```python
from build123d import *

# Parameters (mm, degrees)
F1_DEPTH = 152.4


# Not quite as in the source:
# - ends of sketch curves that miss each other by under 0.0002 mm in the source are joined


with BuildPart() as f1:
    # F0 (on Front) → F1 (new body)
    with BuildSketch(Plane.XZ):
        with BuildLine():
            Line((-8.73125, 3.7119814), (-8.73125, 0.9179814))
            Line((-8.73125, 0.9179814), (-3.96875, 0.9179814))
            Line((-3.96875, 0.9179814), (-3.96875, -7.0195186))
            Line((-3.96875, -7.0195186), (8.73125, -7.0195186))
            Line((8.73125, -7.0195186), (8.73125, -2.0665186))
            ThreePointArc((8.73125, -2.0665186), (5.7032908876, -1.3612616552), (4.438258034, 1.4787376653))
            ThreePointArc((4.438258034, 1.4787376653), (4.3678620463, 1.6652468114), (4.1844976, 1.7434814))
            Line((4.1844976, 1.7434814), (2.06375, 1.7434814))
            ThreePointArc((2.06375, 1.7434814), (1.1469309524, 3.8652258573), (-0.1916191114, 5.7495426677))
            ThreePointArc((-0.1916191114, 5.7495426677), (-4.0073604602, 6.8451953761), (-6.4452349512, 3.7119803958))
            Line((-6.4452349512, 3.7119803958), (-8.73125, 3.7119814))
        make_face()
    extrude(amount=F1_DEPTH)


solid = f1.part
```
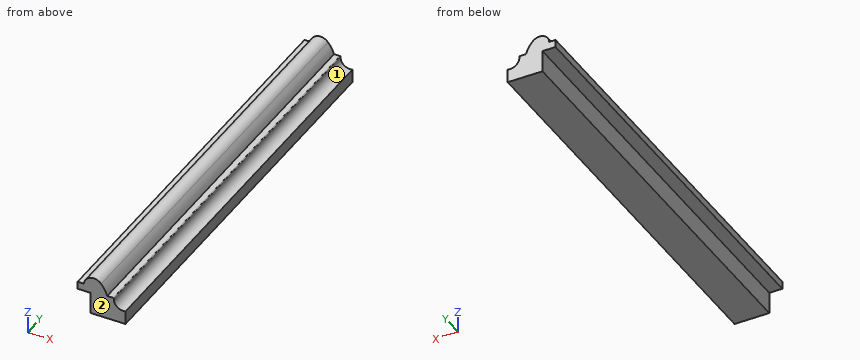
Design review of the part built by this model. Coordinates are the model's own, in mm. Face numbers are marked on the shaded views. Give positions to 0.01 mm unless a question says otherwise; leave off trailing zeros. Write each loop counter-clockwise with the first axis right and the second up, starting at its lowest first coordinate (ties: lowest second). Pieces come first, ordered by that corner, then holes. Notation, with made-up numbers: (10.5, 14) -> (39.5, 14) arc R34 ccw to (39.5, 52) -> close; hole circle Ø7 at (14, 53.5). An arc over 180 degrees is marked (long way). Answer in a Markdown table with one row per item.
(1) To check wall thickness, follow probe 1 along Z at (x, y) = (7, -76.5); probe 2 along X at (y, z) = (-132.5, -2.25); probe 3 along Z at (x, y) = (7.5, -14). State the ranges of each line that lie inside material, in increasing order.
Results:
| item | result |
|---|---|
| probe 1 | -7.02 to -2.04 |
| probe 2 | -3.97 to 8.73 |
| probe 3 | -7.02 to -2.13 |
(2) Consider section C-C (z = -0.75). State the section outline as (x, y) points, then the cut area to 3 significant figures.
Results:
| item | result |
|---|---|
| outline | (-3.97, -152.4) -> (5.12, -152.4) -> (5.12, 0) -> (-3.97, 0) -> close |
| area | 1,390 mm2 |
(3) Clearance check with flat-ended pins moving along their axes: pin 1 (1.1 mm diameter, centred on x = -8, y = -106.5, fed in from +Z); pin 2 (1.4 mm diameter, centred on x = -7.5, y = -76, fed in from -Z); pin 3 (4 mm diameter, centred on y = -55.5, z = -3.5, fed in from -X). State where each tip first meets the part, or that it passes through.
Results:
| item | result |
|---|---|
| pin 1 | z = 3.71 |
| pin 2 | z = 0.92 |
| pin 3 | x = -3.97 |
(4) Consider section A-A (y = -87). State the section outline as (x, z) points, then the cut area to 3 significant figures.
Results:
| item | result |
|---|---|
| outline | (-8.73, 0.92) -> (-3.97, 0.92) -> (-3.97, -7.02) -> (8.73, -7.02) -> (8.73, -2.07) arc R3.49 cw to (4.44, 1.48) arc R0.25 ccw to (4.18, 1.74) -> (2.06, 1.74) arc R11.04 ccw to (-0.19, 5.75) arc R3.54 ccw to (-6.45, 3.71) -> (-8.73, 3.71) -> close |
| area | 140 mm2 |
(5) Mouldability with a two-part tool opening along X and no side actions: class the marked faces 1 and 2 as +X half, -X half, draft (parallel to the pull), parting line (faces both ways), or undercut.
Results:
| item | result |
|---|---|
| face 1 | undercut |
| face 2 | draft |
(6) Consider section B-B (x = -1.5). State the section outline as (y, z) points, then the cut area to 3 significant figures.
Results:
| item | result |
|---|---|
| outline | (-152.4, -7.02) -> (0, -7.02) -> (0, 6.73) -> (-152.4, 6.73) -> close |
| area | 2,090 mm2 |
